Part model, mm, in its own coordinate system. Coordinates: 2 decimals unless noted, no trailing zeros. Order: outer loops, then holes, each group sorted by start corner. A loop starts at its lowest first (then second) coordinate and runs counter-clockwise, first axis right, second up.
1) Cut at B-B (z = 7.5). List the corners of the cut face in (x, y), and give its area (3 significant figures).
2) Cut at A-A (y = 10.25). Give the number of separate pieces and of enclosed holes in the cut face, and give its area (3 significant figures).
3) Pin check, flat tips, straight feed: pin 1 Ø2 at (x, z) = (65.02, 124.79) entering from -Y; pin 2 Ø6 at (x, z) = (114, 45) entering from +Y; pin 3 Ø0.8 at (y, z) = (3.5, 141.5) entering from -X; pin 4 Ø6 at (y, z) = (12.5, 96.5) entering from +X. Stop position of each tip, or through.
4) Cut at C-C (x = 49). List the corners of the cut face in (y, z).
5) Wall check: L1, parallel to Y at x = 94, z = 126.5; L2, parallel to Z at x = 55.5, y = 2.25; L3, parallel to Z at x = 74.5, y = 13.25. Give the ranges that are in metal, low to high.
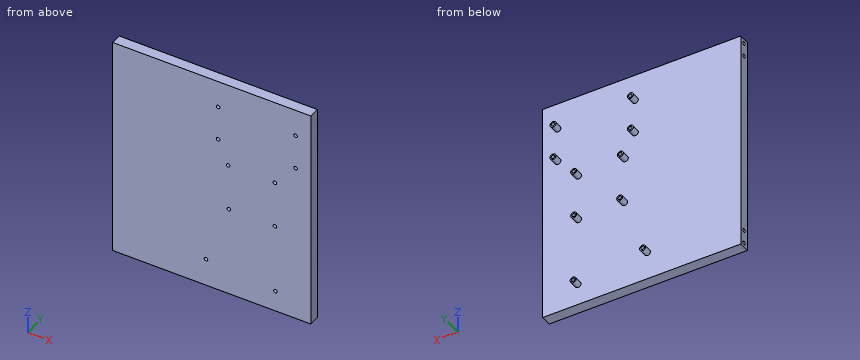
Autodesk Inventor part; units mm, degrees
ref_plane "YZ Plane" through (0, 0, 0) normal (1, 0, 0) x (0, 1, 0)
ref_plane "XZ Plane" through (0, 0, 0) normal (0, 1, 0) x (-1, 0, 0)
ref_plane "XY Plane" through (0, 0, 0) normal (0, 0, 1) x (1, 0, 0)
sketch "Sketch1" plane through (0, 0, 0) normal (0, 1, 0) x (-1, 0, 0)
  line L0 (7.9805, 145.1359) -> (-134.4195, 145.1359)
  line L1 (-134.4195, 145.1359) -> (-134.4195, -21.8641)
  line L2 (-134.4195, -21.8641) -> (7.9805, -21.8641)
  line L3 (7.9805, -21.8641) -> (7.9805, 145.1359)
  line L4 (3.9805, 145.1359) -> (-50.0195, 145.1359)
  line L5 (-50.0195, 145.1359) -> (-50.0195, -21.8641)
  line L6 (-50.0195, -21.8641) -> (3.9805, -21.8641)
  line L7 (3.9805, -21.8641) -> (3.9805, 145.1359)
  line L8 (-126.2985, 137.7454) -> (-60.6985, 137.7454)
  line L9 (-60.6985, 137.7454) -> (-60.6985, 90.7454)
  line L10 (-60.6985, 90.7454) -> (-126.2985, 90.7454)
  line L11 (-126.2985, 90.7454) -> (-126.2985, 137.7454)
  line L12 (-67.0823, 41.9001) -> (-116.0823, 41.9001)
  line L13 (-116.0823, 41.9001) -> (-116.0823, 84.9001)
  line L14 (-116.0823, 84.9001) -> (-67.0823, 84.9001)
  line L15 (-67.0823, 84.9001) -> (-67.0823, 41.9001)
  line L16 (-127.0195, -15.0401) -> (-51.5195, -15.0401)
  line L17 (-51.5195, -15.0401) -> (-51.5195, 38.9599)
  line L18 (-51.5195, 38.9599) -> (-127.0195, 38.9599)
  line L19 (-127.0195, 38.9599) -> (-127.0195, -15.0401)
  circle A0 centre (-55.9195, -1.0401) radius 1.35
  circle A1 centre (-73.0247, 45.9001) radius 1.35
  circle A2 centre (-72.5195, 80.9001) radius 1.35
  circle A3 centre (-107.5195, 45.9001) radius 1.35
  circle A4 centre (-107.5195, 80.9001) radius 1.35
  circle A5 centre (-65.0195, 98.7881) radius 1.35
  circle A6 centre (-65.0195, 124.7881) radius 1.35
  circle A7 centre (-123.0195, 98.7881) radius 1.35
  circle A8 centre (-123.0195, 124.7881) radius 1.35
  circle A9 centre (-106.0195, 35.9599) radius 1.35
  point P0 (0, 0)
  point P1 (-63.2195, -21.8641)
  dimension "d0" = 142.4
  dimension "d1" = 167
  dimension "d2" = 54
  dimension "d3" = 4
  dimension "d21" = 47
  dimension "d22" = 49
  dimension "d23" = 43
  dimension "d25" = 54
  dimension "d27" = 77
  dimension "d29" = 2.7
  dimension "d31" = 14
  dimension "d32" = 71.1
  dimension "d33" = 2.7
  dimension "d34" = 2.7
  dimension "d35" = 2.7
  dimension "d36" = 2.7
  dimension "d52" = 2.7
  dimension "d53" = 2.7
  dimension "d54" = 26
  dimension "d55" = 2.7
  dimension "d56" = 2.7
  dimension "d57" = 26
  dimension "d59" = 58
  dimension "d60" = 15
  dimension "d77" = 2.7
extrude "Extrusion1" add sketch "Sketch1" along normal blind 8 contours L3 L2 L7 L0 | L7 L2 L5 L0 | L5 L2 L1 L0 | L8 L9 L10 L11 | L12 L13 L14 L15 | L19 L18 L17 L16 | A9
sketch "Sketch2" plane through (-7.9805, 0, -21.8641) normal (-1, 0, 0) x (0, 0, 1)
  circle A0 centre (13.5, 4) radius 1.35
  circle A1 centre (153.5, 4) radius 1.35
  line L0 (167, 0) -> (167, 8)
  circle A2 centre (3.5, 4) radius 1.35
  circle A3 centre (163.5, 4) radius 1.35
  point P0 (21.8641, 0)
  dimension "d63" = 2.7
  dimension "d64" = 2.7
  dimension "d65" = 140
  dimension "d67" = 2.7
  dimension "d68" = 2.7
  dimension "d69" = 10
  dimension "d70" = 10
extrude "Extrusion2" cut sketch "Sketch2" against normal blind 8
sketch "Sketch3" plane through (0, 8, 0) normal (0, 1, 0) x (1, 0, 0)
  circle A0 centre (107.9195, 6.0401) radius 1.35
  circle A1 centre (55.9195, 1.0401) radius 1.35
  point P0 (0, 0)
  dimension "d78" = 2.7
  dimension "d79" = 5
  dimension "d80" = 52
extrude "Extrusion3" cut sketch "Sketch3" against normal through all contours A0
sketch "Sketch4" plane through (0, 8, 0) normal (0, 1, 0) x (1, 0, 0)
  circle A0 centre (107.9195, 6.0401) radius 1.35
  circle A1 centre (107.9195, 6.0401) radius 2.25
  circle A2 centre (107.5195, -45.9001) radius 1.35
  circle A3 centre (107.5195, -45.9001) radius 2.25
  circle A4 centre (55.9195, 1.0401) radius 1.35
  circle A5 centre (55.9195, 1.0401) radius 2.25
  circle A6 centre (73.0247, -45.9001) radius 1.35
  circle A7 centre (73.0247, -45.9001) radius 2.25
  circle A8 centre (72.5195, -80.9001) radius 1.35
  circle A9 centre (72.5195, -80.9001) radius 2.25
  circle A10 centre (107.5195, -80.9001) radius 1.35
  circle A11 centre (107.5195, -80.9001) radius 2.25
  circle A12 centre (123.0195, -98.7881) radius 1.35
  circle A13 centre (123.0195, -98.7881) radius 2.25
  circle A14 centre (65.0195, -98.7881) radius 1.35
  circle A15 centre (65.0195, -98.7881) radius 2.25
  circle A16 centre (65.0195, -124.7881) radius 1.35
  circle A17 centre (65.0195, -124.7881) radius 2.25
  circle A18 centre (123.0195, -124.7881) radius 1.35
  circle A19 centre (123.0195, -124.7881) radius 2.25
  circle A20 centre (107.9195, 6.0401) radius 1.35
  circle A21 centre (107.5195, -45.9001) radius 1.35
  circle A22 centre (55.9195, 1.0401) radius 1.35
  circle A23 centre (73.0247, -45.9001) radius 1.35
  circle A24 centre (107.5195, -80.9001) radius 1.35
  circle A25 centre (72.5195, -80.9001) radius 1.35
  circle A26 centre (65.0195, -98.7881) radius 1.35
  circle A27 centre (123.0195, -98.7881) radius 1.35
  circle A28 centre (123.0195, -124.7881) radius 1.35
  circle A29 centre (65.0195, -124.7881) radius 1.35
  point P0 (0, 0)
  dimension "d83" = 4.5
  dimension "d84" = 4.5
  dimension "d85" = 4.5
  dimension "d86" = 4.5
  dimension "d87" = 4.5
  dimension "d88" = 4.5
  dimension "d89" = 4.5
  dimension "d90" = 4.5
  dimension "d91" = 4.5
  dimension "d92" = 4.5
  dimension "d93" = 2.7
  dimension "d94" = 2.7
  dimension "d95" = 2.7
  dimension "d96" = 2.7
  dimension "d97" = 2.7
  dimension "d98" = 2.7
  dimension "d99" = 2.7
  dimension "d100" = 2.7
  dimension "d101" = 2.7
extrude "Extrusion4" add sketch "Sketch4" along normal blind 6
sketch "Sketch5" plane through (-7.9805, 0, -21.8641) normal (-1, 0, 0) x (0, 0, 1)
  line L0 (167, 8) -> (0, 8)
  line L1 (0, 8) -> (167, 8)
  line L2 (167, 8) -> (167, 0)
  line L3 (167, 0) -> (0, 0)
  line L4 (0, 0) -> (0, 8)
  circle A0 centre (13.5, 4) radius 1.35
  circle A1 centre (13.5, 4) radius 1.35
  circle A2 centre (3.5, 4) radius 1.35
  circle A3 centre (3.5, 4) radius 1.35
  circle A4 centre (153.5, 4) radius 1.35
  circle A5 centre (153.5, 4) radius 1.35
  circle A6 centre (163.5, 4) radius 1.35
  circle A7 centre (163.5, 4) radius 1.35
  point P0 (21.8641, 0)
extrude "Extrusion5" add sketch "Sketch5" along normal blind 6
properties part number "house"
Geometry check:
1. outline: (-13.98, 0) - (134.42, 0) - (134.42, 8) - (-13.98, 8) - close
1. area: 1,190 mm2
2. separate pieces: 10
2. enclosed holes: 10
2. area: 102 mm2
3. pin 1: passes through
3. pin 2: stops at y = 8
3. pin 3: stops at x = 0.02
3. pin 4: stops at x = 125.27
4. outline: (0, -21.86) - (8, -21.86) - (8, 145.14) - (0, 145.14) - close
5. L1: y = 0 to 8
5. L2: z = -21.86 to -2.32, 0.24 to 145.14
5. L3: z = 44.2 to 47.6, 79.83 to 81.97
